Geometry check sheet. Reference: drawing and pictorial views, mm from the part's lowest x, y, z. A direction names the side the tool comes from. Coordinates: 2 decimals unless noted, no trailing zeros. Write each loop counter-clockwise with the first axis right and the second up, starting at its lowest first coordinate (ties: lowest second). Pieces come first, ordered by that corner, then holes. Notation, with made-up numbers: (77, 72) -> (92, 72) arc R17 ccw to (92, 80) -> close; hole circle Ø2 at (73, -3.5). An arc over 180 degrees is marked (long way). Put each result on its own line as item: value.
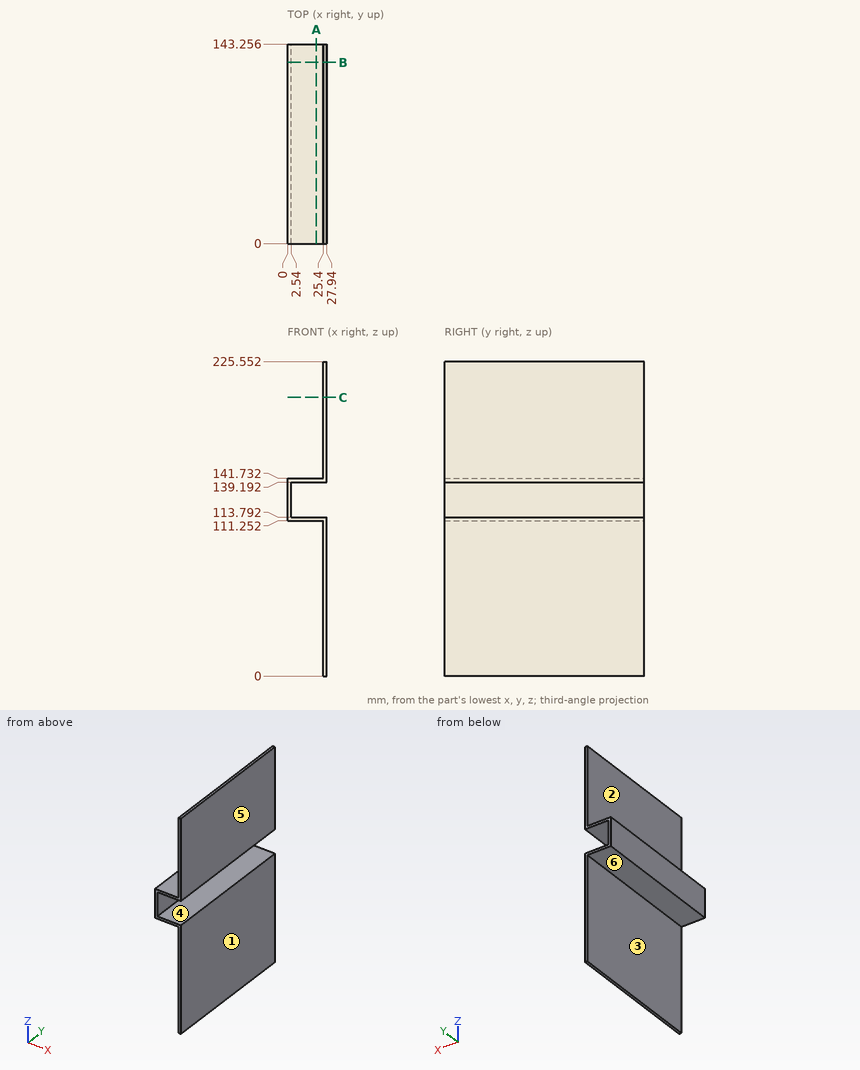
Q1. Cross-section at C-C (z = 200). Record the cut outline in (x, y).
Recorded:
outline: (25.4, 0) -> (27.94, 0) -> (27.94, 143.26) -> (25.4, 143.26) -> close
Q2. Cross-section at A-A (x = 20.5). Record the cut outline in (y, z).
Recorded:
outline: (0, 111.25) -> (143.26, 111.25) -> (143.26, 113.79) -> (0, 113.79) -> close; (0, 139.19) -> (143.26, 139.19) -> (143.26, 141.73) -> (0, 141.73) -> close
Q3. Cross-section at B-B (y = 130). Record the cut outline in (x, z).
Recorded:
outline: (0, 111.25) -> (25.4, 111.25) -> (25.4, 0) -> (27.94, 0) -> (27.94, 113.79) -> (2.54, 113.79) -> (2.54, 139.19) -> (27.94, 139.19) -> (27.94, 225.55) -> (25.4, 225.55) -> (25.4, 141.73) -> (0, 141.73) -> close
Q4. Mould release check, pull along Z, two halves, no side actions. Record for the marked faces 4, 5 and 6: released by +Z, released by -Z, zero draft, split by the parting line, or undercut.
Recorded:
face 4: undercut
face 5: zero draft
face 6: released by -Z
Q5. Depth check by flat-ended pin: P1, Ø4, axis at y = 23, z = 152.5, coming from the -X side; P2, Ø7.5, axis at x = 14, y = 83.5, coming from the +Z side; P3, Ø12.5, axis at x = 16, y = 84, coming from the -Z side. Enter the tip coordinate at first touch or a pass-through.
Recorded:
P1: stops at x = 25.4
P2: stops at z = 141.73
P3: stops at z = 111.25
Q6. Material ranges on line 1 along Z through (x, y) = (14, 98.5); line 2 along Z through (x, y) = (26, 48); line 3 along X through (y, z) = (52.5, 159), recorded low to high.
Recorded:
line 1: z = 111.25 to 113.79, 139.19 to 141.73
line 2: z = 0 to 113.79, 139.19 to 225.55
line 3: x = 25.4 to 27.94
Q7. Tool access check on the marked faces 1, 2 and 3. Record the directions out of +Z, -Z, +X, -X, +Y, -Y that give a thin tool (end or side, any length) a straight path to the whole face; none if there is none.
Recorded:
face 1: +Z, -Z, +X, +Y, -Y
face 2: +Z, -X, +Y, -Y
face 3: -Z, -X, +Y, -Y
